Drawing for the job (mm, zero at the part's lowest x, y, z). Give positions to 0.01 mm unless a question says otherwise; leave off trailing zeros. Write each loop counter-clockwise with the first axis right and the second up, starting at its lowest first coordinate (ties: lowest second). Pieces come first, ordered by that corner, then holes. Notation, with made-up numbers: (32.25, 85.25) - (67.25, 85.25) arc R22 ccw to (67.25, 114.25) - close; hole circle Ø6 at (43, 33.5). An arc over 180 degrees is marked (long way). Answer as a JSON object with one key per item and string values. Group by question number.
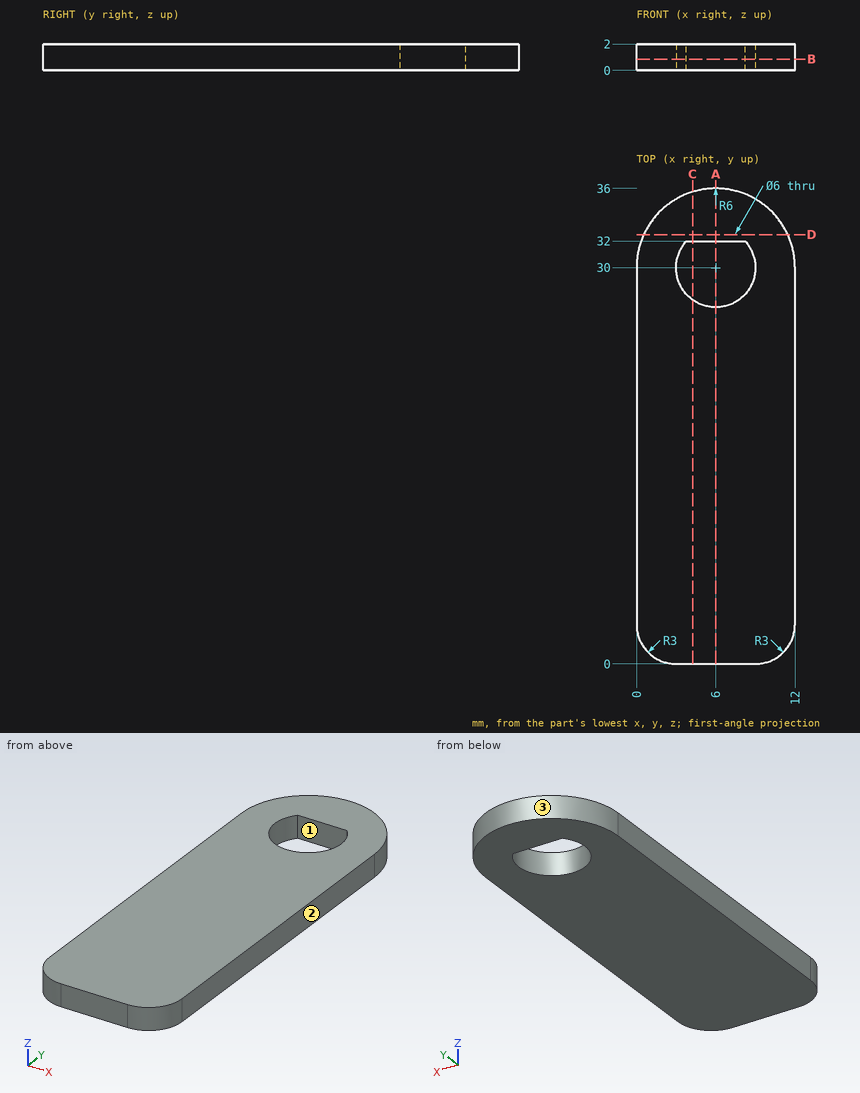
1) Mould opens along Y. For the marked faces 1, 2 and 3 say: pulls with the +Y half, pulls with the -Y half, needs draft (parallel to the pull), parting line crosses it, or undercut.
2) Band-saw the part on A-A (x = 6). List the corners of the cut face in (y, z).
3) Band-saw the part on D-D (y = 32.5). List the corners of the cut face in (x, z), plus the area to 3 significant figures.
4) Probe line 1 (Y direction, x = 6, z = 1.4); line 2 (X direction, y = 30, z = 1); line 3 (Y direction, x = 8.25, z = 1). List the from-to ranges inside material, lowest first.
5) Drop a flat-ended pin along its axis: P1, Ø1, axis at x = 7, z = 1.5, coming from the +Y side. Give the stop position or say it passes through.
6) Band-saw the part on C-C (x = 4.25). List the corners of the cut face in (y, z).
7) Band-saw the part on B-B (z = 0.85). List the corners of the cut face in (x, y).
Verdict:
{
 "1": {"face 1": "undercut", "face 2": "needs draft", "face 3": "pulls with the +Y half"},
 "2": {"outline": "(0, 0) - (27, 0) - (27, 2) - (0, 2) - close; (32, 0) - (36, 0) - (36, 2) - (32, 2) - close"},
 "3": {"outline": "(0.55, 0) - (11.45, 0) - (11.45, 2) - (0.55, 2) - close", "area": "21.8 mm2"},
 "4": {"line 1": "0 to 27, 32 to 36", "line 2": "0 to 3, 9 to 12", "line 3": "0 to 28.02, 31.98 to 35.56"},
 "5": {"P1": "y = 35.98"},
 "6": {"outline": "(0, 0) - (27.56, 0) - (27.56, 2) - (0, 2) - close; (32, 0) - (35.74, 0) - (35.74, 2) - (32, 2) - close"},
 "7": {"outline": "(0, 3) arc R3 ccw to (3, 0) - (9, 0) arc R3 ccw to (12, 3) - (12, 30) arc R6 ccw to (0, 30) - close; hole (3.76, 32) arc R3 ccw (long way) to (8.24, 32) - close"}
}
